The listing builds one solid part. Answer for the finished solid, in the listing's coordinates (mm). A direction names the side the tool comes from. Give positions to 0.01 mm unless a question says otherwise; leave off trailing zeros. Write each loop counter-clockwise with the first axis right and the second up, starting at its lowest first coordinate (ties: lowest second). Pieces come first, ordered by that corner, then holes. Notation, with made-up numbers: (30, -39) - (35, -39) arc R24 ccw to (35, -12) - close; hole circle Ø7 at (20.25, 60). An arc over 180 degrees is marked (long way). Answer as CSV lines item,"result". Start each with the question number.
(1) Straight lines are drawn through the part: probe 1 along Z at (x, y) = (9, 11.9); probe 2 along Y at (x, z) = (0, -2); probe 3 along Y at (x, z) = (-10.5, -2.75). For each, find the intervals that lie inside material, in ascending order.
(2) For faces 1 (the face through (0, -27, 0)), 2 (the face through (16, 0, -8)), 3 (the face through (0, 41, 1)), 4 (the face through (3, 10, -2)), 5 (the face through (0, 27, 0)), determine the directions among +Z, -Z, +X, -X, +Y, -Y from which every point of the face is accessible in a straight line to the end or side of a thin tool.
(3) For a pull along Z with two mould halves and no side action, classify faces 6 (the face through (0, -41, 1)), 7 (the face through (3, 0, -7)), 8 (the face through (7.3, -11.52, -2.93)) as pulls with the +Z half, pulls with the -Z half, needs draft (parallel to the pull), parting line crosses it, or undercut.
(4) Each of these flat-tipped pins is pushed along its axis until it touches: pin 1 Ø8.5 at (x, y) = (-2, 32) entering from -Z; pin 2 Ø4 at (x, z) = (-5, -4.5) entering from +Y; pin 3 Ø6 at (x, y) = (6, -2.5) entering from +Z; pin 4 Ø2.5 at (x, z) = (9, -3) entering from -Y. Where does it stop, or does it pass through?
(5) Find section C-C (x = 0). Write down the section's boundary in (y, z).
(6) Find section B-B (x = 9). Write down the section's boundary in (y, z), then the cut area to 3 significant figures.
(7) Find section A-A (z = -3). Write down the section's boundary in (x, y).
(8) Find section D-D (y = 4.5). Write down the section's boundary in (x, z).
from build123d import *

# Parameters (mm, degrees)
F1_DEPTH = 3
F2_W     = 32
F2_H     = 26
F3_DEPTH = 10
F4_W     = 25.5
F4_H     = 20
F5_DEPTH = 10
F6_R     = 1.7
F7_DEPTH = 101.6


with BuildPart() as f1:
    # F0 (on Top) → F1 (new body)
    with BuildSketch(Plane.XY):
        with BuildLine():
            Line((16, -25), (16, 25))
            ThreePointArc((16, 25), (0, 41), (-16, 25))
            Line((-16, 25), (-16, -25))
            ThreePointArc((-16, -25), (0, -41), (16, -25))
        make_face()
    extrude(amount=F1_DEPTH)

    # F2 (on face) → F3 (join)
    with BuildSketch(Plane(origin=(0, 0, 0), x_dir=(1, 0, 0), z_dir=(0, 0, -1))):
        Rectangle(F2_W, F2_H)
    extrude(amount=F3_DEPTH)

    # F4 (on face) → F5 (cut)
    with BuildSketch(Plane.XY.offset(3)):
        with Locations((3.25, 0)):
            Rectangle(F4_W, F4_H)
    extrude(amount=-F5_DEPTH, mode=Mode.SUBTRACT)

    # F6 (on face) → F7 (cut)
    with BuildSketch(Plane.XZ.offset(13)):
        with Locations((9, -3)):
            Circle(F6_R)
    extrude(amount=-F7_DEPTH, mode=Mode.SUBTRACT)


solid = f1.part
Result set:
1,probe 1,"-10 to -4.7, -1.3 to 3"
1,probe 2,"-13 to -10, 10 to 13"
1,probe 3,"-13 to 13"
2,face 1,"-Z, +X, -X, -Y"
2,face 2,"+Z, -Z, +X, +Y, -Y"
2,face 3,"+Z, -Z, +Y"
2,face 4,"+Z, +X"
2,face 5,"-Z, +X, -X, +Y"
3,face 6,"needs draft"
3,face 7,"pulls with the +Z half"
3,face 8,"undercut"
4,pin 1,"z = 0"
4,pin 2,"y = 13"
4,pin 3,"z = -7"
4,pin 4,"through"
5,outline,"(-41, 0) - (-13, 0) - (-13, -10) - (13, -10) - (13, 0) - (41, 0) - (41, 3) - (10, 3) - (10, -7) - (-10, -7) - (-10, 3) - (-41, 3) - close"
6,outline,"(-38.23, 0) - (-13, 0) - (-13, -1.3) - (-10, -1.3) - (-10, 3) - (-38.23, 3) - close; (-13, -10) - (13, -10) - (13, -4.7) - (10, -4.7) - (10, -7) - (-10, -7) - (-10, -4.7) - (-13, -4.7) - close; (10, -1.3) - (13, -1.3) - (13, 0) - (38.23, 0) - (38.23, 3) - (10, 3) - close"
6,area,"269 mm^2"
7,outline,"(-16, -13) - (7.3, -13) - (7.3, -10) - (-9.5, -10) - (-9.5, 10) - (7.3, 10) - (7.3, 13) - (-16, 13) - close; (10.7, -13) - (16, -13) - (16, -10) - (10.7, -10) - close; (10.7, 10) - (16, 10) - (16, 13) - (10.7, 13) - close"
8,outline,"(-16, -10) - (16, -10) - (16, -7) - (-9.5, -7) - (-9.5, 3) - (-16, 3) - close"
